from build123d import *

# Parameters (mm, degrees)
BOSS_EXTRU_1_DEPTH                             = 30
CONG_1_R                                       = 5
FRAISAGE_POUR_VIS_T_TE_FRAIS_E_M31_D           = 3.4
FRAISAGE_POUR_VIS_T_TE_FRAIS_E_M31_CSINK_D     = 6.3
FRAISAGE_POUR_VIS_T_TE_FRAIS_E_M31_CSINK_ANGLE = 90


with BuildPart() as part:
    # Esquisse1 → Boss.-Extru.1 (new body)
    with BuildSketch(Plane.XY):
        Polygon((-50.2, 0), (50.2, 0), (50.2, -25.3), (75.5, -25.3), (75.5, -20.3), (55.2, -20.3), (55.2, 5), (-55.2, 5), (-55.2, -20.3), (-75.5, -20.3), (-75.5, -25.3), (-50.2, -25.3), align=None)
    extrude(amount=BOSS_EXTRU_1_DEPTH)

    # Congé1
    cong_1_edges = [part.edges().sort_by_distance(p)[0] for p in [
        (-55.2, -20.3, 15),
        (-55.2, 5, 15),
        (55.2, 5, 15),
        (55.2, -20.3, 15),
    ]]
    fillet(cong_1_edges, radius=CONG_1_R)

    # Fraisage pour vis à tête fraisée M31 (through all)
    with Locations(Plane(origin=(0, -20.3, 0), x_dir=(1, 0, 0), z_dir=(0, 1, 0))):
        with Locations((-67.85, -15), (67.85, -15)):
            CounterSinkHole(FRAISAGE_POUR_VIS_T_TE_FRAIS_E_M31_D / 2, FRAISAGE_POUR_VIS_T_TE_FRAIS_E_M31_CSINK_D / 2, counter_sink_angle=FRAISAGE_POUR_VIS_T_TE_FRAIS_E_M31_CSINK_ANGLE)


solid = part.part
Work out the finished part from the listing and answer in its coordinate system (mm). A direction names the side the tool comes from. Give positions to 0.01 mm unless a question says otherwise; leave off trailing zeros. Write each loop counter-clockwise with the first axis right and the second up, starting at its lowest first coordinate (ties: lowest second). Pieces come first, ordered by that corner, then holes.
Q1. For a pull along X with two mould halves and no side action, classify faces 1 (the face through (-55.2, -8, 15)), 2 (the face through (55.2, -8, 15)), 3 (the face through (69.55, -23.55, 14.93)) as released by +X, released by -X, zero draft, split by the parting line, or undercut.
Answer:
face 1: released by -X
face 2: released by +X
face 3: undercut
Q2. The part is cut by section C-C on z = 15. Give the vertices of the cut face in (x, y).
Answer:
outline: (-75.5, -25.3) - (-69.55, -25.3) - (-69.55, -21.75) - (-71, -20.3) - (-75.5, -20.3) - close; (-66.15, -25.3) - (-50.2, -25.3) - (-50.2, 0) - (50.2, 0) - (50.2, -25.3) - (66.15, -25.3) - (66.15, -21.75) - (64.7, -20.3) - (60.2, -20.3) arc R5 cw to (55.2, -15.3) - (55.2, 0) arc R5 ccw to (50.2, 5) - (-50.2, 5) arc R5 ccw to (-55.2, 0) - (-55.2, -15.3) arc R5 cw to (-60.2, -20.3) - (-64.7, -20.3) - (-66.15, -21.75) - close; (69.55, -25.3) - (75.5, -25.3) - (75.5, -20.3) - (71, -20.3) - (69.55, -21.75) - close
Q3. The part is cut by section D-D on z = 24.75. Give the vertices of the cut face in (x, y), and give its area (3 significant figures).
Answer:
outline: (-75.5, -25.3) - (-50.2, -25.3) - (-50.2, 0) - (50.2, 0) - (50.2, -25.3) - (75.5, -25.3) - (75.5, -20.3) - (60.2, -20.3) arc R5 cw to (55.2, -15.3) - (55.2, 0) arc R5 ccw to (50.2, 5) - (-50.2, 5) arc R5 ccw to (-55.2, 0) - (-55.2, -15.3) arc R5 cw to (-60.2, -20.3) - (-75.5, -20.3) - close
area: 1,010 mm2
Q4. The part is cut by section B-B on x = 67.85. Give the vertices of the cut face in (y, z).
Answer:
outline: (-25.3, 0) - (-20.3, 0) - (-20.3, 11.85) - (-21.75, 13.3) - (-25.3, 13.3) - close; (-25.3, 16.7) - (-21.75, 16.7) - (-20.3, 18.15) - (-20.3, 30) - (-25.3, 30) - close
Q5. A tool of negligible diameter and unlimited length cuts with its end or side. For faces 4 (the face through (-1, 0, 15)), 5 (the face through (68, -20.3, 11)), 6 (the face through (-68, -20.3, 11)), 7 (the face through (-75.5, -23, 15)), from which of +Z, -Z, +X, -X, +Y, -Y can it reach the whole face along a straight path? Write none if from no direction.
Answer:
face 4: +Z, -Z, -Y
face 5: +Z, -Z, +X, +Y
face 6: +Z, -Z, -X, +Y
face 7: +Z, -Z, -X, +Y, -Y
Q6. Given pin 1 (4.5 mm diameter, centred on x = 68, z = 17.5, fed in from +Y); pin 2 (12 mm diameter, centred on x = -28, y = -7.5, fed in from +Z); pin 3 (7.5 mm diameter, centred on y = -6.5, z = 8.5, fed in from +X); pin 4 (7.5 mm diameter, centred on y = -13.5, z = 17.5, fed in from -X), each flat-ended and moving along its own axis, determine where each tip first touches the part or whether it passes through.
Answer:
pin 1: stops at y = -20.3
pin 2: passes through
pin 3: stops at x = 55.2
pin 4: stops at x = -55.6
Q7. Straight lines are drawn through the part: L1, parallel to X at y = -24.25, z = 15; L2, parallel to X at y = -12, z = 20.5; L3, parallel to Y at x = 65, z = 19.75. For each, find the intervals that lie inside material, in ascending order.
Answer:
L1: x = -75.5 to -69.55, -66.15 to -50.2, 50.2 to 66.15, 69.55 to 75.5
L2: x = -55.2 to -50.2, 50.2 to 55.2
L3: y = -25.3 to -20.3
Q8. The part is cut by section A-A on y = -6. Give the vertices of the cut face in (x, z).
Answer:
outline: (-55.2, 0) - (-50.2, 0) - (-50.2, 30) - (-55.2, 30) - close; (50.2, 0) - (55.2, 0) - (55.2, 30) - (50.2, 30) - close
